from build123d import *

# Parameters (mm, degrees)
ESQUISSE1_R             = 14
BOSS_EXTRU_1_DEPTH      = 43
CHANFREIN1_SIZE         = 4
ESQUISSE2_R             = 5
BOSS_EXTRU_2_DEPTH      = 6
ESQUISSE3_R             = 1.25
ENL_V_MAT_EXTRU_1_DEPTH = 10
ESQUISSE4_R             = 2.523074606
BOSS_EXTRU_3_DEPTH      = 4
ESQUISSE5_R             = 5.5
BOSS_EXTRU_4_DEPTH      = 7
ESQUISSE6_R             = 4
BOSS_EXTRU_5_DEPTH      = 16


with BuildPart() as part:
    # Esquisse1 → Boss.-Extru.1 (new body)
    with BuildSketch(Plane.XY):
        Circle(ESQUISSE1_R)
    extrude(amount=BOSS_EXTRU_1_DEPTH)

    # Chanfrein1
    chanfrein1_edges = [part.edges().sort_by_distance(p)[0] for p in [
        (-14, 0, 43),
    ]]
    chamfer(chanfrein1_edges, length=CHANFREIN1_SIZE)

    # Esquisse2 → Boss.-Extru.2 (add)
    with BuildSketch(Plane.XY.offset(43)):
        Circle(ESQUISSE2_R)
    extrude(amount=BOSS_EXTRU_2_DEPTH)

    # Esquisse3 → Enlèv. mat.-Extru.1 (cut)
    with BuildSketch(Plane(origin=(0, 0, 0), x_dir=(-1, 0, 0), z_dir=(0, 0, -1))):
        with Locations((0, 9.5)):
            Circle(ESQUISSE3_R)
        with Locations((9.5, 0)):
            Circle(ESQUISSE3_R)
        with Locations((0, -9.5)):
            Circle(ESQUISSE3_R)
        with Locations((-9.5, 0)):
            Circle(ESQUISSE3_R)
    extrude(amount=-ENL_V_MAT_EXTRU_1_DEPTH, mode=Mode.SUBTRACT)

    # Esquisse4 → Boss.-Extru.3 (add)
    with BuildSketch(Plane(origin=(0, 0, 0), x_dir=(-1, 0, 0), z_dir=(0, 0, -1))):
        with Locations(Location((0, 0, 0), (0, 0, 180))):
            Circle(ESQUISSE4_R)
    extrude(amount=BOSS_EXTRU_3_DEPTH)

    # Esquisse5 → Boss.-Extru.4 (add)
    with BuildSketch(Plane(origin=(0, 0, -4), x_dir=(-1, 0, 0), z_dir=(0, 0, -1))):
        Circle(ESQUISSE5_R)
    extrude(amount=BOSS_EXTRU_4_DEPTH)

    # Esquisse6 → Boss.-Extru.5 (add)
    with BuildSketch(Plane(origin=(0, 0, -11), x_dir=(-1, 0, 0), z_dir=(0, 0, -1))):
        Circle(ESQUISSE6_R)
    extrude(amount=BOSS_EXTRU_5_DEPTH)


solid = part.part
Source: CAD feature listing. Evaluate the final solid. Frame: model axes, mm. A direction names the side the tool comes from. Give positions to 0.01 mm unless a question says otherwise; leave off trailing zeros. Write each loop counter-clockwise with the first axis right and the second up, starting at its lowest first coordinate (ties: lowest second). Pieces come first, ordered by that corner, then holes. Notation, with made-up numbers: M 5.25,44.25 L 12.25,44.25 A28 cw 12.25,78.25 Z; hole C -37,-25 d10. An arc over 180 degrees is marked long. Answer as a JSON object with one key per item and string values.
Q1. Cut plane D-D, the plane z = -18. Return the cut outline in (x, y), then the cut area to 3 significant figures.
Geometry check:
{"outline": "C 0,0 d8", "area": "50.3 mm^2"}
Q2. Access query for faces 1 (the face through (-1.86, -1.705, -1.972)), 2 (the face through (0, 0, -27)), 3 (the face through (12.932, -5.362, 19.227)), 4 (the face through (10.75, 0.05, 4.93)), 5 (the face through (-1.08, -4.88, 45.96)). Directions: +Z, -Z, +X, -X, +Y, -Y. A direction counts if a zero-diameter tool reaches every point of the face in a straight line with its end or side. Return the directions, or none.
Geometry check:
{"face 1": "none", "face 2": "-Z, +X, -X, +Y, -Y", "face 3": "+Z, -Z", "face 4": "-Z", "face 5": "+Z"}
Q3. Contact query for flat-ended pins moving along their axis: P1, Ø2, axis at y = 4, z = 2, coming from the +X side; P2, Ø3, axis at x = -9.5, y = 0, coming from the +Z side; P3, Ø0.8, axis at x = 0, y = -10, coming from the -Z side. Output: stop coordinate, or through.
Geometry check:
{"P1": "stops at x = 13.67", "P2": "stops at z = 43", "P3": "stops at z = 10"}
Q4. Cut plane C-C, the plane z = 7.5. Return the cut outline in (x, y), then the cut area to 3 significant figures.
Geometry check:
{"outline": "C 0,0 d28; hole C -9.5,0 d2.5; hole C 0,-9.5 d2.5; hole C 0,9.5 d2.5; hole C 9.5,0 d2.5", "area": "596 mm^2"}
Q5. Ray query, line 1 along Y through (x, z) = (0, 4.5); line 2 along Z through (x, y) = (0.25, 4.25); line 3 along Z through (x, y) = (-9, -3.5). Return the intervals inside material, ascending.
Geometry check:
{"line 1": "y = -14 to -10.75, -8.25 to 8.25, 10.75 to 14", "line 2": "z = -11 to -4, 0 to 49", "line 3": "z = 0 to 43"}
Q6. Mould query, pull axis Y, two halves, no side actions, for faces 6 (the face through (0, 0, 49)), 7 (the face through (0, 10, 10)), 8 (the face through (-9, 0, 10)), 9 (the face through (1.19, -5.37, -7.45)). Classes: +Y half, -Y half, draft (parallel to the pull), parting line (faces both ways), or undercut.
Geometry check:
{"face 6": "draft", "face 7": "undercut", "face 8": "undercut", "face 9": "parting line"}
